from build123d import *

# Parameters (mm, degrees)
SKETCH1_W           = 25
SKETCH1_H           = 48
BOSS_EXTRUDE1_DEPTH = 15
SKETCH2_R           = 3
BOSS_EXTRUDE2_DEPTH = 3


with BuildPart() as part:
    # Sketch1 → Boss-Extrude1 (new body)
    with BuildSketch(Plane(origin=(0, 0, 0), x_dir=(0, 0, -1), z_dir=(1, 0, 0))):
        with Locations((12.5, -24)):
            Rectangle(SKETCH1_W, SKETCH1_H)
    extrude(amount=BOSS_EXTRUDE1_DEPTH)

    # Sketch2 → Boss-Extrude2 (add)
    with BuildSketch(Plane(origin=(0, 0, 0), x_dir=(1, 0, 0), z_dir=(0, 1, 0))):
        with Locations(Location((7.5, 5, 0), (0, 0, 90))):
            Circle(SKETCH2_R)
        Polygon((4.5, 20), (6, 17.401923789), (9, 17.401923789), (10.5, 20), (9, 22.598076211), (6, 22.598076211), align=None)
    extrude(amount=BOSS_EXTRUDE2_DEPTH)


solid = part.part
The model under review builds one solid part; all positions refer to its coordinate system, in mm. A direction names the side the tool comes from. Round coordinates to 2 decimals unless told otherwise and drop trailing zeros. Loops run counter-clockwise (first coordinate to the right, second up) from the corner with the lowest first, then second, coordinate; pieces in that order, holes last. Notation, with made-up numbers: (38.25, -31) -> (95.25, -31) arc R24 ccw to (95.25, 0) -> close; hole circle Ø11 at (80, 75). An arc over 180 degrees is marked (long way). One line per question, with ' | ' between items. Start each with the question number.
Item 1: Add section C-C, the plane z = -5. Write out the cut boundary in (x, y).
Item 2: Wall thickness on line 1 along Y through (x, z) = (10, -23.5): over which ranges is the line inside the solid? List them lowest first. Write a range as [from, to].
Item 3: Add section B-B, the plane z = -20.75. Write out the cut boundary in (x, y), then the cut area to 3 significant figures.
Item 4: For pin 1 (1.5 mm diameter, centred on x = 8, y = 1.5, fed in from -Z); pin 2 (2 mm diameter, centred on x = 12.5, z = -8, fed in from +Y); pin 3 (1.5 mm diameter, centred on x = 7.5, y = 2, fed in from +Z), all flat-tipped, find the tip position at first contact; note any pin that passes through.
Item 5: Draft analysis for pull direction Z (two halves, no side actions). For faces 1 (the face through (9.76, 1.48, -21.28)), 2 (the face through (7, 1, -17.402)), 3 (the face through (7, -48, -12)), state which applies: +Z half, -Z half, draft (parallel to the pull), parting line (faces both ways), or undercut.
Item 6: Add section D-D, the plane x = 3.5. Write out the cut boundary in (y, z).
Item 7: Machinability: for faces 4 (the face through (7, 0, -12)), 5 (the face through (5.24, 1.48, -18.72)), 6 (the face through (8, 1, -22.598)), 7 (the face through (9.74, 1.48, -18.68)), which of the approach directions +Z, -Z, +X, -X, +Y, -Y give a long, thin tool a straight path to every point of the face, cutting with its end or side? Answer none if there is none.
Item 8: Add section A-A, the plane x = 7.5. Write out the cut boundary in (y, z).
Return value:
1) outline: (0, -48) -> (15, -48) -> (15, 0) -> (10.5, 0) -> (10.5, 3) -> (4.5, 3) -> (4.5, 0) -> (0, 0) -> close
2) line 1: y = [-48, 0]
3) outline: (0, -48) -> (15, -48) -> (15, 0) -> (10.07, 0) -> (10.07, 3) -> (4.93, 3) -> (4.93, 0) -> (0, 0) -> close | area: 735 mm2
4) pin 1: stops at z = -22.6 | pin 2: stops at y = 0 | pin 3: stops at z = -2
5) face 1: -Z half | face 2: undercut | face 3: draft
6) outline: (-48, -25) -> (0, -25) -> (0, 0) -> (-48, 0) -> close
7) face 4: +Y | face 5: -X, +Y | face 6: -Z, +X, -X, +Y | face 7: +X, +Y
8) outline: (-48, -25) -> (0, -25) -> (0, -22.6) -> (3, -22.6) -> (3, -17.4) -> (0, -17.4) -> (0, -8) -> (3, -8) -> (3, -2) -> (0, -2) -> (0, 0) -> (-48, 0) -> close
